Can you work these out from the model? Positions are in its coordinate system, mm. Face numbers are marked on the shaded views. A direction names the side the tool comes from. Coordinates: 2 decimals unless noted, no trailing zeros. Loops run counter-clockwise (first coordinate to the right, second up) from the corner with the lowest first, then second, coordinate; pieces in that order, holes last. Notation, with made-up numbers: M -13,-25 L 18,-25 A22 ccw 18,4 Z; hole C 28,58.25 d4. An arc over 180 degrees is marked long. Answer as a JSON object with one key per item and string values. Group by question number.
Item 1: I'm going to push flat-ended pins straight in: pin 1 Ø1 at (x, y) = (1.5, 2) entering from +Z; pin 2 Ø8 at (x, z) = (-4, 7) entering from -Y; pin 3 Ø3 at (x, y) = (7.5, 0) entering from +Z; pin 4 Ø1 at (y, z) = (5.5, -1) entering from -X. Where does each tip first touch, or does it pass through?
Item 2: If I drill on line 1 (Y direction, x = -2.75, z = 7); line 2 (Z direction, x = 0, y = -2.75); line 3 (X direction, y = 3.25, z = -3.75), over which ranges is the centre line in solid material (lowest first)?
Item 3: Suppose I cut it at D-D (y = -2.75). Write out the boundary of the cut face in (x, z).
Item 4: Suppose I cut it at B-B (y = 6.75). Write out the boundary of the cut face in (x, z).
Item 5: Suppose I cut it at A-A (z = 0). Write out the boundary of the cut face in (x, y).
Item 6: Suppose I cut it at C-C (x = 0). Write out the boundary of the cut face in (y, z), then the cut area to 3 significant figures.
Item 7: We'd pull the mould along X, two halves only. Please class the marked faces 1, 2 and 3: +X half, -X half, draft (parallel to the pull), parting line (faces both ways), or undercut.
Item 8: Which directions (+Z, -Z, +X, -X, +Y, -Y) give clear straight access to the entire face, cutting with the end or side of a thin tool? Please do the marked faces 4, 5 and 6.
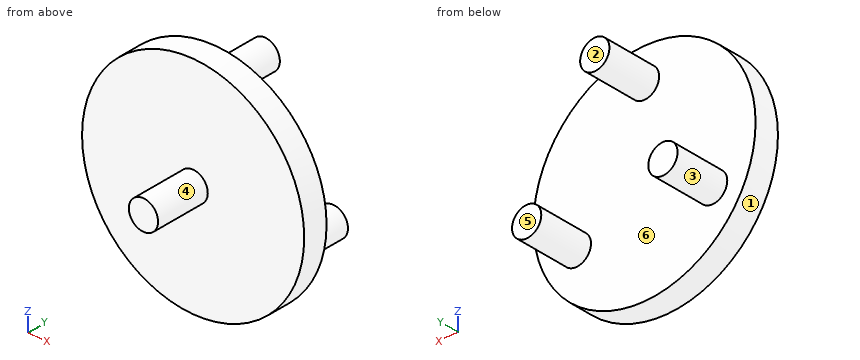
```python
from build123d import *

# Parameters (mm, degrees)
F0_R     = 12
F1_DEPTH = 1.35
F2_R     = 1.58
F3_DEPTH = 6
F4_R     = 1.58
F5_DEPTH = 6


with BuildPart() as f1:
    # F0 (on Front) → F1 (new body, symmetric)
    with BuildSketch(Plane.XZ):
        Circle(F0_R)
    extrude(amount=F1_DEPTH, both=True)

    # F2 (on face) → F3 (join)
    with BuildSketch(Plane.XZ.offset(1.35)):
        Circle(F2_R)
    extrude(amount=F3_DEPTH)

    # F4 (on face) → F5 (join)
    with BuildSketch(Plane(origin=(0, 1.35, 0), x_dir=(-1, 0, 0), z_dir=(0, 1, 0))):
        with Locations((0, 8.5)):
            Circle(F4_R)
        with Locations((-7.3612159322, -4.25)):
            Circle(F4_R)
        with Locations((7.3612159322, -4.25)):
            Circle(F4_R)
    extrude(amount=F5_DEPTH)


solid = f1.part
```
From the geometry:
{
 "1": {"pin 1": "z = 9.72", "pin 2": "y = -1.35", "pin 3": "z = 10.39", "pin 4": "through"},
 "2": {"line 1": "-1.35 to 1.35", "line 2": "-1.58 to 1.58", "line 3": "-8.86 to -5.86, 5.86 to 8.86"},
 "3": {"outline": "C 0,0 d3.16"},
 "4": {"outline": "C -7.36,-4.25 d3.16; C 0,8.5 d3.16; C 7.36,-4.25 d3.16"},
 "5": {"outline": "M -12,-1.35 L -1.58,-1.35 L -1.58,-7.35 L 1.58,-7.35 L 1.58,-1.35 L 12,-1.35 L 12,1.35 L -12,1.35 Z"},
 "6": {"outline": "M -7.35,-1.58 L -1.35,-1.58 L -1.35,-12 L 1.35,-12 L 1.35,6.92 L 7.35,6.92 L 7.35,10.08 L 1.35,10.08 L 1.35,12 L -1.35,12 L -1.35,1.58 L -7.35,1.58 Z", "area": "103 mm2"},
 "7": {"face 1": "parting line", "face 2": "draft", "face 3": "undercut"},
 "8": {"face 4": "-Y", "face 5": "+Z, -Z, +X, -X, +Y", "face 6": "+Y"}
}
